Input: part model. Units: mm. Frame: model coordinates. A direction names the side the tool comes from. Give positions to 0.01 mm unless a question says otherwise; leave off trailing zeros. Order: outer loops, then holes, each group sorted by start corner. A loop starts at its lowest first (then second) coordinate and runs counter-clockwise, first axis right, second up. Notation, with made-up numbers: (51.25, 76.5) - (108.25, 76.5) arc R18 cw to (108.25, 81.5) - close; hole circle Ø1 at (-1, 79). An arc over 180 degrees is marked (long way). Answer in a Markdown table with one row per item. Add a question column.
from build123d import *

# Parameters (mm, degrees)
EXTRUDE_1_DEPTH     = 17
SKETCH_2_R          = 0.6
CUT_EXTRUDE_1_DEPTH = 1
CHAMFER_1_SIZE      = 1
CHAMFER_1_SIZE2     = 0.839099631


with BuildPart() as part:
    # Эскиз1 → Бобышка-Вытянуть1 (new body)
    with BuildSketch(Plane(origin=(0, 0, 0), x_dir=(1, 0, 0), z_dir=(0, 1, 0))):
        Polygon((3, 0), (-3, 0), (-3, 1.567384684), (-1, 2.5), (1, 2.5), (3, 1.567384684), align=None)
    extrude(amount=EXTRUDE_1_DEPTH)

    # Эскиз2 → Вырез-Вытянуть1 (cut)
    with BuildSketch(Plane.XY):
        with Locations((0, 2.35)):
            Circle(SKETCH_2_R)
        with Locations((0, 14.3)):
            Circle(SKETCH_2_R)
    extrude(amount=-CUT_EXTRUDE_1_DEPTH, mode=Mode.SUBTRACT)

    # Фаска1
    chamfer_1_edges = [part.edges().sort_by_distance(p)[0] for p in [
        (-0.6, 2.35, 0),
        (-0.6, 14.3, 0),
    ]]
    chamfer_1_side = [part.faces().sort_by_distance(p)[0] for p in [
        (0, 8.503968803, 0),
    ]]
    chamfer(chamfer_1_edges, length=CHAMFER_1_SIZE, length2=CHAMFER_1_SIZE2, reference=chamfer_1_side[0])


solid = part.part
Q1. Access query for faces 4 (the flat face through (0, 0, -1)), 5 (the flat face through (0, 14, -1)). Directions: +Z, -Z, +X, -X, +Y, -Y. A direction counts if a zero-diameter tool reaches every point of the face in a straight line with its end or side. Return the directions, or none.
Q2. Section B-B, the plane y = 2.35. Return loops of the section in (x, z), then the cut area to 3 significant figures.
Q3. Section A-A, the plane x = 0. Return loops of the section in (y, z), then the cut area to 3 significant figures.
Q4. Line query: probe 1 along Y at (x, z) = (-0.2, -0.3); probe 2 along Y at (x, z) = (0, -0.9); probe 3 along X at (y, z) = (1.5, -0.45). Output: solid intervals per line, ascending.
Q5. Section C-C, the plane z = -0.3. Return loops of the section in (x, y), then the cut area to 3 significant figures.
Q6. Contact query for flat-ended pins moving along their axis: P1, Ø1, axis at x = 0, y = 2.5, coming from the +Z side; P2, Ø0.6, axis at x = -0.5, y = 14.5, coming from the +Z side; P3, Ø1.6, axis at x = 0, y = 2.35, coming from the +Z side. Output: stop coordinate, or through.
Q7. Pull-direction query (Y, two-part tool) for faces 1 (the flat face through (1.99, 8.38, -2.04)), 2 (the flat face through (0, 2, -1)), 3 (the flat face through (0, 17, -1)); classes: +Y half, -Y half, draft (parallel to the pull), parting line (faces both ways), or undercut.
Q8. Section D-D, the plane y = 10.5. Return loops of the section in (x, z), then the cut area to 3 significant figures.
Computed:
| question | item | result |
|---|---|---|
| 1 | face 4 | +Z, -Z, +X, -X, -Y |
| 1 | face 5 | +Z |
| 2 | outline | (-3, -1.57) - (-1, -2.5) - (1, -2.5) - (3, -1.57) - (3, 0) - (1.6, 0) - (0.6, -0.84) - (0.6, -1) - (-0.6, -1) - (-0.6, -0.84) - (-1.6, 0) - (-3, 0) - close |
| 2 | area | 11.1 mm^2 |
| 3 | outline | (0, -2.5) - (17, -2.5) - (17, 0) - (15.9, 0) - (14.9, -0.84) - (14.9, -1) - (13.7, -1) - (13.7, -0.84) - (12.7, 0) - (3.95, 0) - (2.95, -0.84) - (2.95, -1) - (1.75, -1) - (1.75, -0.84) - (0.75, 0) - (0, 0) - close |
| 3 | area | 38.4 mm^2 |
| 4 | probe 1 | y = 0 to 1.12, 3.58 to 13.07, 15.53 to 17 |
| 4 | probe 2 | y = 0 to 1.75, 2.95 to 13.7, 14.9 to 17 |
| 4 | probe 3 | x = -3 to -0.64, 0.64 to 3 |
| 5 | outline | (-3, 0) - (3, 0) - (3, 17) - (-3, 17) - close; hole circle Ø2.48 at (0, 2.35); hole circle Ø2.48 at (0, 14.3) |
| 5 | area | 92.3 mm^2 |
| 6 | P1 | stops at z = -0.8 |
| 6 | P2 | stops at z = -0.64 |
| 6 | P3 | stops at z = -0.67 |
| 7 | face 1 | draft |
| 7 | face 2 | undercut |
| 7 | face 3 | +Y half |
| 8 | outline | (-3, -1.57) - (-1, -2.5) - (1, -2.5) - (3, -1.57) - (3, 0) - (-3, 0) - close |
| 8 | area | 13.1 mm^2 |
